Here's how the part is built. I have some questions about the finished solid (model axes, mm). Face numbers are marked on the shaded views. A direction names the side the tool comes from. Coordinates: 2 decimals unless noted, no trailing zeros. Write each loop counter-clockwise with the first axis right and the second up, starting at its lowest first coordinate (ties: lowest second). Pieces come first, ordered by that corner, then holes.
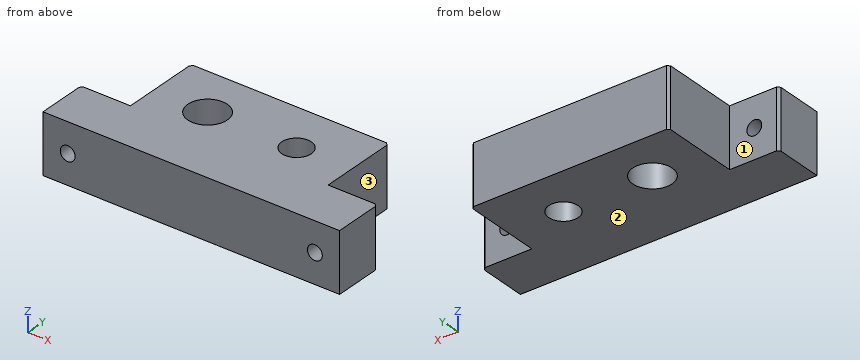
from build123d import *

# Parameters (mm, degrees)
F0_R          = 4
F0_R_2        = 3
F1_DEPTH      = 6
F1_DEPTH_BACK = 6
F2_R          = 1.5
F3_DEPTH      = 26.001
F4_SIZE       = 0.5


with BuildPart() as f1:
    # F0 (on Top) → F1 (new body, two sides)
    with BuildSketch(Plane.XY) as f1_sk:
        Polygon((-30, 10), (-30, 0), (30, 0), (30, 10), (20, 10), (20, 26), (-20, 26), (-20, 10), align=None)
        with Locations((-9, 16)):
            Circle(F0_R, mode=Mode.SUBTRACT)
        with Locations((9, 16)):
            Circle(F0_R_2, mode=Mode.SUBTRACT)
    extrude(amount=F1_DEPTH)
    extrude(f1_sk.sketch, amount=-F1_DEPTH_BACK)

    # F2 (on face) → F3 (cut, through all)
    with BuildSketch(Plane.XZ):
        with Locations((-25, 0)):
            Circle(F2_R)
        with Locations((25, 0)):
            Circle(F2_R)
    extrude(amount=-F3_DEPTH, mode=Mode.SUBTRACT)

    # F4
    f4_edges = [f1.edges().sort_by_distance(p)[0] for p in [
        (-20, 26, 0),
        (20, 26, 0),
        (30, 10, 0),
        (-30, 10, 0),
    ]]
    chamfer(f4_edges, length=F4_SIZE)


solid = f1.part
1. On a 3-axis mill with a long thin cutter (end or side, diameter ignored), from which of +Z, -Z, +X, -X, +Y, -Y can I reach the whole of each face in a straight line? I mean the marked faces 1, 2 and 3. Say none if no direction works.
2. I want a section at B-B (y = 16). List the corners of the cut face in (x, z) for me.
3. If I drill on line 1 (X direction, y = 13.5, z = -0.5); line 2 (Y direction, x = 9, z = -4.25); line 3 (Z direction, x = 25, y = 4.25), over which ranges is the centre line in solid material (lowest first)?
4. I want a section at D-D (x = 25). List the corners of the cut face in (y, z) for me, then the cut area to 3 significant figures.
5. I want a section at C-C (z = 5). List the corners of the cut face in (x, y) for me.
6. For pin 1 Ø3.5 at (x, y) = (9, 16) entering from -Z; pin 2 Ø4 at (y, z) = (20.5, -2.5) entering from -X; pin 3 Ø5 at (x, z) = (-24.5, 1) entering from +Y; pin 4 Ø1 at (y, z) = (21.5, 0.5) entering from +X, each with a flat end and sliding along its axis, tell me the tip position at first contact or that it passes through.
7. I want a section at A-A (x = -9). List the corners of the cut face in (y, z) for me, then the cut area to 3 significant figures.
Response values:
1. face 1: +Z, -Z, -X, +Y
1. face 2: -Z, +X, -X, +Y, -Y
1. face 3: +Z, -Z, +X, +Y
2. outline: (-20, -6) - (-13, -6) - (-13, 6) - (-20, 6) - close; (-5, -6) - (6, -6) - (6, 6) - (-5, 6) - close; (12, -6) - (20, -6) - (20, 6) - (12, 6) - close
3. line 1: x = -20 to -12.12, -5.88 to 7.34, 10.66 to 20
3. line 2: y = 0 to 13, 19 to 26
3. line 3: z = -6 to -1.5, 1.5 to 6
4. outline: (0, -6) - (10, -6) - (10, -1.5) - (0, -1.5) - close; (0, 1.5) - (10, 1.5) - (10, 6) - (0, 6) - close
4. area: 90.0 mm2
5. outline: (-30, 0) - (30, 0) - (30, 9.5) - (29.5, 10) - (20, 10) - (20, 25.5) - (19.5, 26) - (-19.5, 26) - (-20, 25.5) - (-20, 10) - (-29.5, 10) - (-30, 9.5) - close; hole circle Ø8 at (-9, 16); hole circle Ø6 at (9, 16)
6. pin 1: passes through
6. pin 2: stops at x = -20
6. pin 3: stops at y = 10
6. pin 4: stops at x = 20
7. outline: (0, -6) - (12, -6) - (12, 6) - (0, 6) - close; (20, -6) - (26, -6) - (26, 6) - (20, 6) - close
7. area: 216 mm2
